from build123d import *

# Parameters (mm, degrees)
F1_DEPTH = 5
F3_DEPTH = 1.9
F3_TAPER = 10
F5_DEPTH = 1
F6_W     = 8
F6_H     = 3.4583588084
F7_DEPTH = 25
F8_W     = 14.479
F8_H     = 1
F9_DEPTH = 25


with BuildPart() as f1:
    # F0 (on Front) → F1 (new body)
    with BuildSketch(Plane.XZ):
        Polygon((0, 5), (0, 0), (0, -1.2), (10.4, -1.2), (10.4, 0), (10.4, 5), (9.2, 5), (9.2, 0), (1.2, 0), (1.2, 5), align=None)
    extrude(amount=F1_DEPTH)

    # F2 (on face) → F3 (join)
    with BuildSketch(Plane.XY):
        with BuildLine():
            ThreePointArc((5.9758246596, -2.5), (5.7485908778, -1.9514091222), (5.2, -1.7241753404))
            Line((5.2, -1.7241753404), (5.2, -3.2758246596))
            ThreePointArc((5.2, -3.2758246596), (5.7485908778, -3.0485908778), (5.9758246596, -2.5))
        make_face()
        with BuildLine():
            Line((5.2, -3.2758246596), (5.2, -1.7241753404))
            ThreePointArc((5.2, -1.7241753404), (4.4241753404, -2.5), (5.2, -3.2758246596))
        make_face()
    extrude(amount=F3_DEPTH, taper=F3_TAPER)

    # F4 (on face) → F5 (join)
    with BuildSketch(Plane(origin=(0, 0, 0), x_dir=(-1, 0, 0), z_dir=(0, 1, 0))):
        with BuildLine():
            ThreePointArc((-4.45, 0.320197377), (-3.2557777905, 1.1928752721), (-2.8, 2.6))
            ThreePointArc((-2.8, 2.6), (-3.5029437252, 4.2970562748), (-5.2, 5))
            ThreePointArc((-5.2, 5), (-7.5697601456, 2.9797852714), (-5.95, 0.320197377))
            ThreePointArc((-5.95, 0.320197377), (-5.2, 0.2), (-4.45, 0.320197377))
        make_face()
        with BuildLine():
            Line((-4.45, 0), (-4.45, 0.320197377))
            ThreePointArc((-4.45, 0.320197377), (-5.2, 0.2), (-5.95, 0.320197377))
            Line((-5.95, 0.320197377), (-5.95, 0))
            Line((-5.95, 0), (-4.45, 0))
        make_face()
    extrude(amount=-F5_DEPTH)

    # F6 (on face) → F7 (cut)
    with BuildSketch(Plane.XY):
        with Locations((5.2, -3.2708205958)):
            Rectangle(F6_W, F6_H)
    extrude(amount=F7_DEPTH, mode=Mode.SUBTRACT)

    # F8 (on face) → F9 (cut)
    with BuildSketch(Plane.XY.offset(5)):
        with Locations((3.1605, -4.5)):
            Rectangle(F8_W, F8_H)
    extrude(amount=-F9_DEPTH, mode=Mode.SUBTRACT)


solid = f1.part
Work out the finished part from the listing and answer in its coordinate system (mm). A direction names the side the tool comes from. Give positions to 0.01 mm unless a question says otherwise; leave off trailing zeros. Loops run counter-clockwise (first coordinate to the right, second up) from the corner with the lowest first, then second, coordinate; pieces in that order, holes last. Notation, with made-up numbers: (12.25, -21) -> (56.25, -21) arc R26 ccw to (56.25, 10) -> close; hole circle Ø5 at (-10, -20.75). An arc over 180 degrees is marked (long way). Use a Markdown table: item, result. Add a question column.
1. Section C-C on z = 2.25 is taken. Determine the outline of the cut face in (x, y).
2. Find the intervals of material crossed by probe 1 along X at (y, z) = (-3, 0.75); probe 2 along X at (y, z) = (-0.45, 3); probe 3 along Y at (x, z) = (5, 0.25), in increasing order.
3. Section D-D on x = 8.25 is taken. Determine the outline of the cut face in (y, z).
4. Determine the mould class of faces 1 (the flat face through (10, -2, 5)), 2 (the flat face through (0, -2, 2)), 3 (the flat face through (1.2, -2, 2)) for opening direction X: released by +X, released by -X, zero draft, split by the parting line, or undercut.
5. A flat-ended cylindrical pin translates along its axis: pin 1 Ø1.2 at (x, y) = (7, -2) entering from +Z. Find the tip coordinate at first contact, or state that the pin passes through.
6. For faces 4 (the flat face through (9.2, -2, 3)), 5 (the flat face through (5, -1, 3)), 6 (the flat face through (5, -2, -1.2)), determine the directions among +Z, -Z, +X, -X, +Y, -Y from which every point of the face is accessible in a straight line to the end or side of a thin tool.
7. Section B-B on y = -0.45 is taken. Determine the outline of the cut face in (x, z), and give its area (3 significant figures).
8. Section A-A on x = 7 is taken. Determine the outline of the cut face in (y, z).
Results below:
| question | item | result |
|---|---|---|
| 1 | outline | (0, -4) -> (1.2, -4) -> (1.2, 0) -> (0, 0) -> close; (2.83, -1) -> (7.57, -1) -> (7.57, 0) -> (2.83, 0) -> close; (9.2, -4) -> (10.4, -4) -> (10.4, 0) -> (9.2, 0) -> close |
| 2 | probe 1 | x = 0 to 1.2, 9.2 to 10.4 |
| 2 | probe 2 | x = 0 to 1.2, 2.83 to 7.57, 9.2 to 10.4 |
| 2 | probe 3 | y = -1 to 0 |
| 3 | outline | (-4, -1.2) -> (0, -1.2) -> (0, 0) -> (-4, 0) -> close |
| 4 | face 1 | zero draft |
| 4 | face 2 | released by -X |
| 4 | face 3 | undercut |
| 5 | pin 1 | stops at z = 0 |
| 6 | face 4 | +Z, +Y, -Y |
| 6 | face 5 | +Z, -Y |
| 6 | face 6 | -Z, +X, -X, +Y, -Y |
| 7 | outline | (0, -1.2) -> (10.4, -1.2) -> (10.4, 5) -> (9.2, 5) -> (9.2, 0) -> (5.95, 0) -> (5.95, 0.32) arc R2.4 ccw (long way) to (4.45, 0.32) -> (4.45, 0) -> (1.2, 0) -> (1.2, 5) -> (0, 5) -> close |
| 7 | area | 42.9 mm^2 |
| 8 | outline | (-4, -1.2) -> (0, -1.2) -> (0, 0) -> (-4, 0) -> close; (-1, 1.01) -> (0, 1.01) -> (0, 4.19) -> (-1, 4.19) -> close |
